from build123d import *

# Parameters (mm, degrees)
F0_W     = 45
F0_H     = 20.5
F1_DEPTH = 1.6
F2_R     = 8
F3_DEPTH = 4
F4_DEPTH = 3.9878


with BuildPart() as f1:
    # F0 (on Front) → F1 (new body)
    with BuildSketch(Plane.XZ):
        Rectangle(F0_W, F0_H)
    extrude(amount=F1_DEPTH)

    # F2 (on face) → F3 (join)
    with BuildSketch(Plane.XZ.offset(1.6)):
        with Locations((-13.5, 0)):
            Circle(F2_R)
    extrude(amount=F3_DEPTH)

    # F2 (on face) → F4 (join)
    with BuildSketch(Plane.XZ.offset(1.6)):
        with BuildLine():
            ThreePointArc((21.5, 0), (13.5, 8), (5.5, 0))
            ThreePointArc((5.5, 0), (13.5, -8), (21.5, 0))
        make_face()
    extrude(amount=F4_DEPTH)


solid = f1.part
Part model, mm, in its own coordinate system. A direction names the side the tool comes from. Give positions to 0.01 mm unless a question says otherwise; leave off trailing zeros. Order: outer loops, then holes, each group sorted by start corner. A loop starts at its lowest first (then second) coordinate and runs counter-clockwise, first axis right, second up. Notation, with made-up numbers: (20, -32) - (77, -32) arc R7 ccw to (77, -24) - close; hole circle Ø9 at (69, 8.25). An arc over 180 degrees is marked (long way). Use a Markdown table: item, result.
1) Saw through at B-B on z = -5. List the corners of the cut face in (x, y) (3 decimals).
Checked values:
| item | result |
|---|---|
| outline | (-22.5, -1.6) - (-19.745, -1.6) - (-19.745, -5.6) - (-7.255, -5.6) - (-7.255, -1.6) - (7.255, -1.6) - (7.255, -5.588) - (19.745, -5.588) - (19.745, -1.6) - (22.5, -1.6) - (22.5, 0) - (-22.5, 0) - close |
2) 3-axis set-ups, long thin cutter, end or side, ignore diameter. For faces 1 (the flat face through (-22.5, -1, 0)), 2 (the cylindrical face through (-15.23, -3.57, -7.81)): which of +Z, -Z, +X, -X, +Y, -Y reach the whole face in a straight line?
Checked values:
| item | result |
|---|---|
| face 1 | +Z, -Z, -X, +Y, -Y |
| face 2 | -Y |
3) Saw through at C-C on y = -3.9. List the corners of the cut face in (x, z), plus the area to 3 significant figures.
Checked values:
| item | result |
|---|---|
| outline | circle Ø16 at (-13.5, 0); circle Ø16 at (13.5, 0) |
| area | 402 mm² |
4) Saw through at A-A on x = -13.5. List the corners of the cut face in (y, z).
Checked values:
| item | result |
|---|---|
| outline | (-5.6, -8) - (-1.6, -8) - (-1.6, -10.25) - (0, -10.25) - (0, 10.25) - (-1.6, 10.25) - (-1.6, 8) - (-5.6, 8) - close |
5) Flat gauge pins, fed straight in: P1, Ø4, axis at x = -14, z = 5, coming from the +Y side; P2, Ø2, axis at x = -10, y = -4.5, coming from the +Z side; P3, Ø6, axis at x = 11, z = 1.5, coming from the -Y side; P4, Ø1.5, axis at y = -4.5, z = -0.5, coming from the +X side. Where does each tip first touch, or does it go through?
Checked values:
| item | result |
|---|---|
| P1 | y = 0 |
| P2 | z = 7.6 |
| P3 | y = -5.59 |
| P4 | x = 21.5 |
6) Two-plate mould, pull along X, no slides. Class faces 3 (the cylindrical face through (15.23, -3.57, 7.81)), 4 (the flat face through (22.5, -1, 0)), 5 (the flat face through (0, -1, -10.25)), 6 (the flat face through (0, -1.6, 0)): +X half, -X half, draft (parallel to the pull), parting line (faces both ways), or undercut.
Checked values:
| item | result |
|---|---|
| face 3 | undercut |
| face 4 | +X half |
| face 5 | draft |
| face 6 | undercut |
7) Saw through at D-D on x = 13.5. List the corners of the cut face in (y, z), plus the area to 3 significant figures.
Checked values:
| item | result |
|---|---|
| outline | (-5.59, -8) - (-1.6, -8) - (-1.6, -10.25) - (0, -10.25) - (0, 10.25) - (-1.6, 10.25) - (-1.6, 8) - (-5.59, 8) - close |
| area | 96.6 mm² |
8) Probe L1, parallel to Y at x = 1.5, z = -8.75; L2, parallel to X at y = -3.35, z = -7; L3, parallel to X at y = -2.75, z = 2. List the from-to ranges inside material, lowest first. Write a range as from..to.
Checked values:
| item | result |
|---|---|
| L1 | -1.6..0 |
| L2 | -17.37..-9.63, 9.63..17.37 |
| L3 | -21.25..-5.75, 5.75..21.25 |
